Source: CAD feature listing. Evaluate the final solid. Frame: model axes, mm. Round coordinates to 2 decimals unless told otherwise and drop trailing zeros. Loops run counter-clockwise (first coordinate to the right, second up) from the corner with the lowest first, then second, coordinate; pieces in that order, holes last.
(1) Section C-C, the plane y = -2.25. Return the cut outline in (x, z) (3 decimals), plus the area to 3 significant figures.
(2) Section A-A, the plane x = 7.5. Return the cut outline in (y, z) (3 decimals), plus the area to 3 significant figures.
(3) Section B-B, the plane z = 23.61. Return the cut outline in (x, y).
(4) Mould query, pull axis Z, two halves, no side actions, for faces 1 (the cylindrical face through (8.281, -7.395, 81.455)), 2 (the flat face through (7, -7, 120)), 3 (the flat face through (15, -8, 59)), 4 (the cylindrical face through (5.918, -7.395, 21.547)). Classes: pulls with the +Z half, pulls with the -Z half, needs draft (parallel to the pull), parting line crosses it, or undercut.
(5) Material intervals for probe 1 along X at (y, z) = (-7.25, 96.37); probe 2 along Z at (x, y) = (5.5, -7.25); probe 3 along X at (y, z) = (-10, 94), sorted ascending.
```python
from build123d import *

# Parameters (mm, degrees)
SKETCH_1_W          = 15
SKETCH_1_H          = 15
EXTRUDE_1_DEPTH     = 120
SKETCH_2_R          = 2.6
CUT_EXTRUDE_1_DEPTH = 122.86057607


with BuildPart() as part:
    # 草图1 → 凸台-拉伸1 (new body)
    with BuildSketch(Plane.XY):
        with Locations((7.5, -7.5)):
            Rectangle(SKETCH_1_W, SKETCH_1_H)
    extrude(amount=EXTRUDE_1_DEPTH)

    # 草图2 → 切除-拉伸1 (cut, through all)
    with BuildSketch(Plane(origin=(0, 0, 0), x_dir=(1, 0, 0), z_dir=(0, 1, 0))):
        with Locations(Location((7.5, -23.61, 0), (0, 0, 270))):
            Circle(SKETCH_2_R)
        with Locations(Location((7.5, -96.37, 0), (0, 0, 270))):
            Circle(SKETCH_2_R)
        with Locations(Location((7.5, -41.025, 0), (0, 0, 270))):
            Circle(SKETCH_2_R)
        with Locations(Location((7.5, -78.975, 0), (0, 0, 270))):
            Circle(SKETCH_2_R)
    extrude(amount=-CUT_EXTRUDE_1_DEPTH, mode=Mode.SUBTRACT)


solid = part.part
```
Output values:
1. outline: (0, 0) - (15, 0) - (15, 120) - (0, 120) - close; hole circle Ø5.2 at (7.5, 23.61); hole circle Ø5.2 at (7.5, 41.025); hole circle Ø5.2 at (7.5, 78.975); hole circle Ø5.2 at (7.5, 96.37)
1. area: 1,720 mm2
2. outline: (-15, 0) - (0, 0) - (0, 21.01) - (-15, 21.01) - close; (-15, 26.21) - (0, 26.21) - (0, 38.425) - (-15, 38.425) - close; (-15, 43.625) - (0, 43.625) - (0, 76.375) - (-15, 76.375) - close; (-15, 81.575) - (0, 81.575) - (0, 93.77) - (-15, 93.77) - close; (-15, 98.97) - (0, 98.97) - (0, 120) - (-15, 120) - close
2. area: 1,490 mm2
3. outline: (0, -15) - (4.9, -15) - (4.9, 0) - (0, 0) - close; (10.1, -15) - (15, -15) - (15, 0) - (10.1, 0) - close
4. face 1: undercut
4. face 2: pulls with the +Z half
4. face 3: needs draft
4. face 4: undercut
5. probe 1: x = 0 to 4.9, 10.1 to 15
5. probe 2: z = 0 to 21.95, 25.27 to 39.36, 42.69 to 77.31, 80.64 to 94.71, 98.03 to 120
5. probe 3: x = 0 to 6.43, 8.57 to 15
